Part model, mm, in its own coordinate system. A direction names the side the tool comes from. Round coordinates to 2 decimals unless told otherwise and drop trailing zeros. Loops run counter-clockwise (first coordinate to the right, second up) from the corner with the lowest first, then second, coordinate; pieces in that order, holes last. Notation, with made-up numbers: (52.5, 11) - (110.5, 11) arc R13 cw to (110.5, 21) - close; hole circle Ø4 at (76.5, 63). An arc over 180 degrees is marked (long way). Write each question's results on one line, items separated by ' | '. Start each with the question number.
(1) Cut at C-C, the plane y = 6. List the corners of the cut face in (x, z).
(2) Flat gauge pins, fed straight in: P1, Ø3, axis at x = -135, y = 4.5, coming from the -Z side; P2, Ø5, axis at x = -132, y = 4.5, coming from the -Z side. Where does each tip first touch, or does it go through?
(3) Cut at D-D, the plane z = -23.5. List the corners of the cut face in (x, y).
(4) Drill centre lines: L1, parallel to Z at x = -46, y = 2; L2, parallel to Z at x = 19, y = 1.5; L3, parallel to X at y = 7.5, z = 81. Where is each one in solid material? Low to high.
(5) Mould opens along X. For faces 1 (the face through (-114, 10, 79)), 2 (the face through (215.026, 4.93, 85.215)), 3 (the face through (12.2, 4.9, -8.8)) say: released by +X, released by -X, zero draft, split by the parting line, or undercut.
(6) Cut at A-A, the plane z = 6. List the corners of the cut face in (x, y), then the cut area to 3 significant figures.
(7) Tool access for faces 4 (the face through (-114, 0, 79)), 5 (the face through (-70.363, 4.93, 10.434)): list every direction of +Z, -Z, +X, -X, +Y, -Y with a clear straight run to the whole face (end or side of a thin tool).
(8) Cut at B-B, the plane x = -151. List the corners of the cut face in (y, z), then the cut area to 3 significant figures.
Autodesk Inventor part; units mm, degrees
ref_plane "YZ Plane" through (0, 0, 0) normal (1, 0, 0) x (0, 1, 0)
ref_plane "XZ Plane" through (0, 0, 0) normal (0, 1, 0) x (-1, 0, 0)
ref_plane "XY Plane" through (0, 0, 0) normal (0, 0, 1) x (1, 0, 0)
sketch "Sketch3" plane through (0, 0, 0) normal (0, 1, 0) x (-1, 0, 0)
  line L0 (-219.2412, 70.0717) -> (200.7588, -89.9283)
  line L1 (205.7588, -63.9283) -> (-110.8967, 62.7339)
  line L2 (200.7588, -89.9283) -> (310.7588, -89.9283)
  line L3 (278.7588, -63.9283) -> (205.7588, -63.9283)
  line L4 (278.7588, 86.3746) -> (278.7588, -63.9283)
  line L5 (310.7588, -89.9283) -> (310.7588, 190.0717)
  line L6 (-110.8967, 86.3746) -> (278.7588, 86.3746)
  line L7 (278.7588, 112.3746) -> (-110.8967, 112.3746)
  line L8 (-110.8967, 150.1531) -> (278.7588, 150.1531)
  line L9 (278.7588, 150.1531) -> (278.7588, 112.3746)
  line L10 (-339.2412, 190.0717) -> (310.7588, 190.0717)
  line L11 (-110.8967, 112.3746) -> (-110.8967, 150.1531)
  line L12 (-339.2412, 70.0717) -> (-219.2412, 70.0717)
  line L13 (-339.2412, 70.0717) -> (-339.2412, 190.0717)
  circle A0 centre (-256.9912, 109.3217) radius 3.25
  circle A1 centre (-256.9912, 85.8217) radius 3.25
  circle A2 centre (-231.2412, 90.3217) radius 17
  circle A3 centre (-205.4912, 85.8217) radius 3.25
  circle A4 centre (-205.4912, 109.3217) radius 3.25
  line L14 (-110.8967, 86.3746) -> (-110.8967, 62.7339)
  line L15 (260, -45.1696) -> (209.3714, -45.1696)
  line L16 (209.3714, -45.1696) -> (-72.5921, 67.6158)
  line L17 (-72.5921, 67.6158) -> (260, 67.6158)
  line L18 (260, 67.6158) -> (260, -45.1696)
  line L19 (260, 131.1334) -> (-92.1379, 131.1334)
  line L20 (-92.1379, 131.1334) -> (-92.1379, 131.3943)
  line L21 (-92.1379, 131.3943) -> (260, 131.3943)
  line L22 (260, 131.3943) -> (260, 131.1334)
  point P0 (0, 0)
extrude "Extrusion2" add sketch "Sketch3" along normal blind 10 contours L12 L13 L10 L5 L2 L0 | L1 L14 L6 L4 L3 | L7 L11 L8 L9
sketch "Sketch4" plane through (-310.7588, 0, -89.9283) normal (-1, 0, 0) x (0, 0, 1)
  line L0 (0, 0) -> (280, 0)
  line L1 (280, 0) -> (280, 10)
  line L2 (0, 10) -> (280, 10)
  line L3 (0, 0) -> (0, 10)
  point P0 (89.9283, 0)
extrude "Extrusion3" add sketch "Sketch4" along normal blind 100
properties part number "YFlanPlate" material "Aluminum 6061"
A:
1) outline: (-410.76, -89.93) - (-200.76, -89.93) - (219.24, 70.07) - (339.24, 70.07) - (339.24, 190.07) - (-410.76, 190.07) - close; hole (-260, -45.17) - (-209.37, -45.17) - (72.59, 67.62) - (-260, 67.62) - close; hole (-260, 131.13) - (92.14, 131.13) - (92.14, 131.39) - (-260, 131.39) - close; hole circle Ø6.5 at (205.49, 85.82); hole circle Ø6.5 at (205.49, 109.32); hole circle Ø34 at (231.24, 90.32); hole circle Ø6.5 at (256.99, 85.82); hole circle Ø6.5 at (256.99, 109.32)
2) P1: z = -65.45 | P2: z = -64.69
3) outline: (-410.76, 0) - (-260, 0) - (-260, 10) - (-410.76, 10) - close; (-155.2, 0) - (-26.38, 0) - (-26.38, 10) - (-155.2, 10) - close
4) L1: -30.97 to 20.18, 67.62 to 131.13, 131.39 to 190.07 | L2: -6.21 to 46.18, 67.62 to 131.13, 131.39 to 190.07 | L3: -410.76 to 217.02, 245.46 to 339.24
5) face 1: zero draft | face 2: undercut | face 3: released by +X
6) outline: (-410.76, 0) - (-260, 0) - (-260, 10) - (-410.76, 10) - close; (-81.45, 0) - (51.05, 0) - (51.05, 10) - (-81.45, 10) - close | area: 2,830 mm2
7) face 4: +Z, -Z, +X, -X, -Y | face 5: +Y, -Y
8) outline: (0, -70.97) - (10, -70.97) - (10, -21.82) - (0, -21.82) - close; (0, 67.62) - (10, 67.62) - (10, 131.13) - (0, 131.13) - close; (0, 131.39) - (10, 131.39) - (10, 190.07) - (0, 190.07) - close | area: 1,710 mm2
